Geometry check sheet. Reference: the model listing, model coordinates, mm. Round coordinates to 2 decimals unless told otherwise and drop trailing zeros. Order: outer loops, then holes, each group sorted by start corner. A loop starts at its lowest first (then second) coordinate and runs counter-clockwise, first axis right, second up. Notation, with made-up numbers: (39, -37.75) - (92, -37.75) arc R27 ccw to (92, -7.75) - close; hole circle Ø3 at (35, 72.25). An arc over 180 degrees is marked (long way). Use a Markdown table: item, result. Add a question column.
(1) Section check C-C on x = 208.5. Record the boundary of the cut face in (y, z).
(2) Thickness scan on line 1 along X through (y, z) = (87.5, 4.5); line 2 along X through (y, z) = (85.5, 4.75). Record the ranges inside material, lowest first. Write a range as [from, to].
(3) Section check B-B on y = 49. Record the boundary of the cut face in (x, z).
(4) Section check A-A on z = 1.25. Record the boundary of the cut face in (x, y).
(5) Gauge pin test, flat end, axial feed: P1, Ø1.5, axis at y = 40, z = 5, coming from the -X side. Record the tip position at first contact, or that the pin passes through.
Autodesk Inventor part; units mm, degrees
ref_plane "YZ Plane" through (0, 0, 0) normal (1, 0, 0) x (0, 1, 0)
ref_plane "XZ Plane" through (0, 0, 0) normal (0, 1, 0) x (-1, 0, 0)
ref_plane "XY Plane" through (0, 0, 0) normal (0, 0, 1) x (1, 0, 0)
sketch "Sketch1" plane through (0, 0, 0) normal (0, 0, 1) x (1, 0, 0)
  line L0 (0, 0) -> (190.5, 0)
  arc A0 (190.5, 0) -> (215.4067, 20.4187) centre (190.5, 25.4) ccw
  line L1 (215.4067, 20.4187) -> (228.1067, 83.9187)
  arc A1 (228.1067, 83.9187) -> (203.2, 114.3) centre (203.2, 88.9) ccw
  line L2 (203.2, 114.3) -> (0, 114.3)
  line L3 (0, 114.3) -> (0, 0)
  dimension "d4" = 25.4
  dimension "d5" = 25.4
  dimension "d6" = 228.6
  dimension "d9" = 114.3
extrude "Extrusion1" add sketch "Sketch1" along normal blind 6.35
properties part number "ImprintPart1"
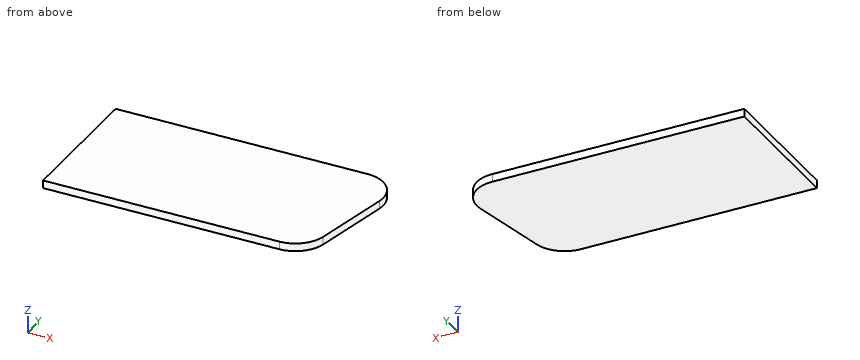
Check sheet entries:
| question | item | result |
|---|---|---|
| 1 | outline | (7.48, 0) - (113.74, 0) - (113.74, 6.35) - (7.48, 6.35) - close |
| 2 | line 1 | x = [0, 228.56] |
| 2 | line 2 | x = [0, 228.37] |
| 3 | outline | (0, 0) - (221.12, 0) - (221.12, 6.35) - (0, 6.35) - close |
| 4 | outline | (0, 0) - (190.5, 0) arc R25.4 ccw to (215.41, 20.42) - (228.11, 83.92) arc R25.4 ccw to (203.2, 114.3) - (0, 114.3) - close |
| 5 | P1 | stops at x = 0 |
